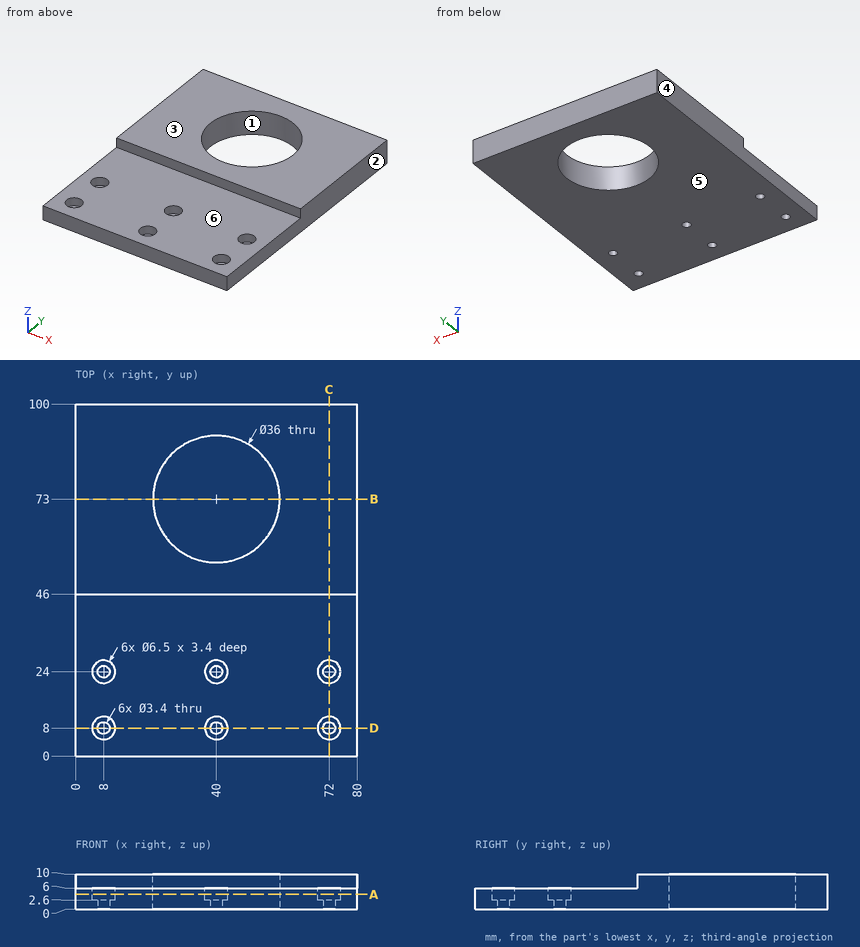
The drawing under review shows one solid part. Ordinate dimensions are in mm from its lowest x, y, z. A direction names the side the tool comes from. Round coordinates to 2 decimals unless told otherwise and drop trailing zeros. Loops run counter-clockwise (first coordinate to the right, second up) from the corner with the lowest first, then second, coordinate; pieces in that order, holes last. Notation, with made-up numbers: (37, 65.5) - (70, 65.5) arc R18 ccw to (70, 98.5) - close; hole circle Ø9 at (47, 58). An arc over 180 degrees is marked (long way). Use a Markdown table: item, result. Add a question column.
Q1. Add section C-C (x = 72). State the section outline as (y, z) points.
Q2. Add section D-D (y = 8). State the section outline as (x, z) points.
Q3. Insertion check: pin 1 Ø7 at (x, y) = (7, 23.5) entering from +Z; pin 2 Ø6 at (x, y) = (72, 24) entering from +Z; pin 3 Ø1.2 at (x, z) = (24, 8) entering from -Y. Each pin has a flat end and moves straight along its axis. Give the tip position at first contact, or say it passes through.
Q4. For probe 1 along Y at (x, z) = (40, 4.9); probe 2 along Y at (x, z) = (8, 5.2); probe 3 along Y at (x, z) = (40, 1.6), list the stretches that pass through material, from the lowest coordinate up.
Q5. Add section B-B (y = 73). State the section outline as (x, z) points, plus the area to 3 significant figures.
Q6. Add section A-A (z = 4.25). State the section outline as (x, y) points, plus the area to 3 significant figures.
Q7. Machinability: for the marked faces 5 and 6, which of the approach directions +Z, -Z, +X, -X, +Y, -Y give a long, thin tool a straight path to every point of the face, cutting with its end or side? Answer none if there is none.
Q8. The part is to be moulded in two halves that separate along X. For the marked faces 1, 2, 3 and 4, say which applies: pulls with the +X half, pulls with the -X half, needs draft (parallel to the pull), parting line crosses it, or undercut.
Worked answers:
| question | item | result |
|---|---|---|
| 1 | outline | (0, 0) - (6.3, 0) - (6.3, 2.6) - (4.75, 2.6) - (4.75, 6) - (0, 6) - close; (9.7, 0) - (22.3, 0) - (22.3, 2.6) - (20.75, 2.6) - (20.75, 6) - (11.25, 6) - (11.25, 2.6) - (9.7, 2.6) - close; (25.7, 0) - (100, 0) - (100, 10) - (46, 10) - (46, 6) - (27.25, 6) - (27.25, 2.6) - (25.7, 2.6) - close |
| 2 | outline | (0, 0) - (6.3, 0) - (6.3, 2.6) - (4.75, 2.6) - (4.75, 6) - (0, 6) - close; (9.7, 0) - (38.3, 0) - (38.3, 2.6) - (36.75, 2.6) - (36.75, 6) - (11.25, 6) - (11.25, 2.6) - (9.7, 2.6) - close; (41.7, 0) - (70.3, 0) - (70.3, 2.6) - (68.75, 2.6) - (68.75, 6) - (43.25, 6) - (43.25, 2.6) - (41.7, 2.6) - close; (73.7, 0) - (80, 0) - (80, 6) - (75.25, 6) - (75.25, 2.6) - (73.7, 2.6) - close |
| 3 | pin 1 | z = 6 |
| 3 | pin 2 | z = 2.6 |
| 3 | pin 3 | y = 46 |
| 4 | probe 1 | 0 to 4.75, 11.25 to 20.75, 27.25 to 55, 91 to 100 |
| 4 | probe 2 | 0 to 4.75, 11.25 to 20.75, 27.25 to 100 |
| 4 | probe 3 | 0 to 6.3, 9.7 to 22.3, 25.7 to 55, 91 to 100 |
| 5 | outline | (0, 0) - (22, 0) - (22, 10) - (0, 10) - close; (58, 0) - (80, 0) - (80, 10) - (58, 10) - close |
| 5 | area | 440 mm² |
| 6 | outline | (0, 0) - (80, 0) - (80, 100) - (0, 100) - close; hole circle Ø6.5 at (8, 8); hole circle Ø6.5 at (8, 24); hole circle Ø36 at (40, 73); hole circle Ø6.5 at (40, 8); hole circle Ø6.5 at (40, 24); hole circle Ø6.5 at (72, 8); hole circle Ø6.5 at (72, 24) |
| 6 | area | 6,780 mm² |
| 7 | face 5 | -Z, +X, -X, +Y, -Y |
| 7 | face 6 | +Z, +X, -X, -Y |
| 8 | face 1 | undercut |
| 8 | face 2 | pulls with the +X half |
| 8 | face 3 | needs draft |
| 8 | face 4 | pulls with the -X half |
